Could you check a few things on this model? Use its own coordinates, in mm. A direction names the side the tool comes from. Round coordinates to 2 decimals unless told otherwise and drop trailing zeros. Write each question's results on one line, items separated by ' | '.
Autodesk Inventor part; units mm, degrees
ref_plane "dummy_XY" through (7, -4, 0) normal (1, 0, 0) x (0, 0, -1)
ref_plane "dummy_YZ" through (7, -4, 0) normal (0, 0, -1) x (0, 1, 0)
ref_plane "dummy_ZX" through (7, -4, 0) normal (0, 1, 0) x (1, 0, 0)
sketch "Sketch_11" plane through (0, 0, 0) normal (1, 0, 0) x (0, 1, 0)
  line L0 (5, 7.5) -> (4.1225, 7.5)
  arc A0 (0.9321, 7.25) -> (4.1225, 7.5) centre (2.5175, 7.5) ccw
  line L1 (0.9321, 7.25) -> (0.25, 7.25)
  line L2 (0.25, 7.25) -> (0, 7.5)
  line L3 (0, 7.5) -> (-3.5, 7.5)
  line L4 (-3.5, 7.5) -> (-4, 7)
  line L5 (-4, 7) -> (-4, -6.9999)
  line L6 (-4, -6.9999) -> (-3.5, -7.5)
  line L7 (-3.5, -7.5) -> (0, -7.5)
  line L8 (0, -7.5) -> (0.25, -7.25)
  line L9 (0.25, -7.25) -> (0.9321, -7.25)
  arc A1 (4.1225, -7.5) -> (0.9321, -7.25) centre (2.5175, -7.5) ccw
  line L10 (4.1225, -7.5) -> (5, -7.5)
  line L11 (5, -7.5) -> (5.5, -7)
  line L12 (5.5, -7) -> (5.5, 7)
  line L13 (5.5, 7) -> (5, 7.5)
extrude "Extrusion1" add sketch "Sketch_11" along normal blind 294
sketch "Sketch_17" plane through (0, 0, 0) normal (0, 0, 1) x (1, 0, 0)
  line L0 (7, -4.5) -> (7, 6)
  line L1 (7, 6) -> (10, 6)
  line L2 (10, 6) -> (10, 1)
  line L3 (10, 1) -> (8.75, 1)
  line L4 (8.75, 1) -> (8.75, -4.5)
  line L5 (8.75, -4.5) -> (7, -4.5)
  line L6 (7, -4.5) -> (7, 6)
revolve "Revolution1" cut sketch "Sketch_17" angle 360 about axis through (7, -4.5, 0) along (0, -1, 0)
pattern_linear "Rectangular Pattern1" count 8 spacing 40 along (1, 0, 0) of "Revolution1"
ref_plane "dummy_XY" through (7, -4, 0) normal (1, 0, 0) x (0, 0, -1)
ref_plane "dummy_YZ" through (7, -4, 0) normal (0, 0, -1) x (0, 1, 0)
ref_plane "dummy_ZX" through (7, -4, 0) normal (0, 1, 0) x (1, 0, 0)
ref_plane "slider_XY" through (20, 0, 0) normal (-1, 0, 0) x (0, 0, -1)
ref_plane "slider_YZ" through (20, 0, 0) normal (0, 0, -1) x (0, -1, 0)
ref_plane "slider_ZX" through (20, 0, 0) normal (0, -1, 0) x (-1, 0, 0)
ref_plane "slider2_XY" through (100, 0, 0) normal (-1, 0, 0) x (0, 0, -1)
ref_plane "slider2_YZ" through (100, 0, 0) normal (0, 0, -1) x (0, -1, 0)
ref_plane "slider2_ZX" through (100, 0, 0) normal (0, -1, 0) x (-1, 0, 0)
properties part number "LU15AL294K2720100_rail"
1) If we mould it in two halves opening along Z, with no side actions, what happens to faces 3 (the flat face through (145, -4, 0)), 4 (the flat face through (167, 1, -2)), 5 (the flat face through (49, 1, 0))? For each: released by +Z, released by -Z, zero draft, split by the parting line, or undercut.
Model answer:
face 3: zero draft | face 4: undercut | face 5: undercut
2) For faces 1 (the flat face through (0, 1, 0)), 2 (the cylindrical face through (244, 3, 0)), which set-ups out of +Z, -Z, +X, -X, +Y, -Y let a thin tool reach every point of the face, with its end or its side?
Model answer:
face 1: +Z, -Z, -X, +Y, -Y | face 2: +Y
3) I'm going to push flat-ended pins straight in: pin 1 (1.5 mm diameter, centred on x = 167.5, y = 2.5, fed in from -Z); pin 2 (1.8 mm diameter, centred on x = 8.5, z = 0.5, fed in from +Y). Where does each tip first touch, or does it pass through?
Model answer:
pin 1: stops at z = -6.09 | pin 2: stops at y = 1
4) I need wall thicknesses on line 1 (Z direction, x = 167, y = 2.95); line 2 (Z direction, x = 207, y = 2.45); line 3 (Y direction, x = 247.5, z = -1.75). Which ranges of each line are inside material? Lowest first, please.
Model answer:
line 1: z = -5.95 to -3, 3 to 5.95 | line 2: z = -5.9 to -3, 3 to 5.9 | line 3: y = -4 to 1
